Build history of the part. All positions in model axes, mm. A direction names the side the tool comes from. Give positions to 0.01 mm unless a question says otherwise; leave off trailing zeros. Loops run counter-clockwise (first coordinate to the right, second up) from the corner with the lowest first, then second, coordinate; pieces in that order, holes last.
1) Two-plate mould, pull along X, no slides. Class faces 4 (the cylindrical face through (-19.32, 3.89, 2.79)), 5 (the flat face through (0, -12.5, 2)), 6 (the flat face through (-25, 0, 2)): +X half, -X half, draft (parallel to the pull), parting line (faces both ways), or undercut.
2) 3-axis set-ups, long thin cutter, end or side, ignore diameter. For faces 1 (the flat face through (25, 0, 2)), 2 (the cylindrical face through (-19.36, -3.93, 2.79)), 3 (the cylindrical face through (0.249, 2.965, 6.199)): which of +Z, -Z, +X, -X, +Y, -Y reach the whole face in a straight line?
3) Flat gauge pins, fed straight in: P1, Ø4, axis at x = -4.5, y = 7.5, coming from the +Z side; P2, Ø1.5, axis at y = 6.5, z = 5, coming from the +X side; P3, Ø1.5, axis at x = -0.5, y = 7.5, coming from the +Z side. Where does each tip first touch, or does it go through?
4) Band-saw the part on B-B on z = 0.5. State how many separate pieces and enclosed holes the cut face has, then the cut area to 3 significant figures.
5) Band-saw the part on A-A on x = -2.5. List the corners of the cut face in (y, z).
6) Wall check: line 1 (Y direction, x = -0.5, z = 1); line 2 (Y direction, x = 19.5, z = 0.5); line 3 (X direction, y = -3.5, z = 0.5). Give the ranges that are in metal, low to high.
```python
from build123d import *

# Parameters (mm, degrees)
F0_W     = 50
F0_H     = 25
F0_W_2   = 40
F0_H_2   = 4.5
F1_DEPTH = 6.5
F2_R     = 5
F3_R     = 2.24999
F4_R     = 1
F5_R     = 3


# Not quite as in the source:
# - a fillet or chamfer is up to 0.001 mm smaller than in the source, because OpenCascade refuses the exact size


with BuildPart() as f1:
    # F0 (on Top) → F1 (new body)
    with BuildSketch(Plane.XY):
        Rectangle(F0_W, F0_H)
        with Locations((0, -5.5)):
            Rectangle(F0_W_2, F0_H_2, mode=Mode.SUBTRACT)
        with Locations((0, 5.5)):
            Rectangle(F0_W_2, F0_H_2, mode=Mode.SUBTRACT)
    extrude(amount=F1_DEPTH)

    # F2
    f2_edges = [f1.edges().sort_by_distance(p)[0] for p in [
        (-25, -12.5, 3.25),
        (25, -12.5, 3.25),
        (25, 12.5, 3.25),
        (-25, 12.5, 3.25),
    ]]
    fillet(f2_edges, radius=F2_R)

    # F3 (radius 2.25 in the source; OpenCascade refuses exactly that, so slightly less here)
    f3_edges = [f1.edges().sort_by_distance(p)[0] for p in [
        (-20, -3.25, 3.25),
        (-20, -7.75, 3.25),
        (-20, 3.25, 3.25),
        (-20, 7.75, 3.25),
        (20, -7.75, 3.25),
        (20, -3.25, 3.25),
        (20, 3.25, 3.25),
        (20, 7.75, 3.25),
    ]]
    fillet(f3_edges, radius=F3_R)

    # F4
    f4_edges = [f1.edges().sort_by_distance(p)[0] for p in [
        (0, -7.75, 6.5),
        (0, 3.25, 6.5),
    ]]
    fillet(f4_edges, radius=F4_R)

    # F5
    f5_edges = [f1.edges().sort_by_distance(p)[0] for p in [
        (25, 0, 6.5),
    ]]
    fillet(f5_edges, radius=F5_R)


solid = f1.part
```
Findings below:
1. face 4: undercut
1. face 5: draft
1. face 6: -X half
2. face 1: +Z, -Z, +X, +Y, -Y
2. face 2: +Z, -Z
2. face 3: +Z
3. P1: stops at z = 6.5
3. P2: stops at x = 24.9
3. P3: stops at z = 6.37
4. separate pieces: 1
4. enclosed holes: 2
4. area: 877 mm2
5. outline: (-12.5, 0) - (-7.75, 0) - (-7.75, 5.5) arc R1 ccw to (-8.75, 6.5) - (-9.5, 6.5) arc R3 ccw to (-12.5, 3.5) - close; (-3.25, 0) - (3.25, 0) - (3.25, 5.5) arc R1 ccw to (2.25, 6.5) - (-2.25, 6.5) arc R1 ccw to (-3.25, 5.5) - close; (7.75, 0) - (12.5, 0) - (12.5, 3.5) arc R3 ccw to (9.5, 6.5) - (8.75, 6.5) arc R1 ccw to (7.75, 5.5) - close
6. line 1: y = -12.5 to -7.75, -3.25 to 3.25, 7.75 to 12.5
6. line 2: y = -12.5 to -6.91, -4.09 to 4.09, 6.91 to 12.5
6. line 3: x = -25 to -18.78, 18.78 to 25
